from build123d import *
from OCP.BRepFilletAPI import BRepFilletAPI_MakeChamfer

# Parameters (mm, degrees)
SKETCH1_R           = 25
BOSS_EXTRUDE1_DEPTH = 140.711096
SKETCH2_R           = 14.171797432
CUT_EXTRUDE1_DEPTH  = 146.084845995
CHAMFER1_SIZE       = 2.459659
CHAMFER1_SIZE2      = 1.420085


with BuildPart() as part:
    # Sketch1 → Boss-Extrude1 (new body)
    with BuildSketch(Plane(origin=(0, 0, 0), x_dir=(1, 0, 0), z_dir=(0, 1, 0))):
        with Locations(Location((0, 0, 0), (0, 0, 270))):
            Circle(SKETCH1_R)
    extrude(amount=BOSS_EXTRUDE1_DEPTH)

    # Sketch2 → Cut-Extrude1 (cut, through all)
    with BuildSketch(Plane(origin=(0, 0, 0), x_dir=(1, 0, 0), z_dir=(0, 1, 0))):
        with Locations(Location((0, 0, 0), (0, 0, 270))):
            Circle(SKETCH2_R)
    extrude(amount=CUT_EXTRUDE1_DEPTH, mode=Mode.SUBTRACT)

    # Chamfer1: one chamfer whose edges measure the first distance from different faces: ONE call of the kernel's chamfer builder (chamfer() names one face for all edges)
    chamfer1_edges_1 = [part.edges().sort_by_distance(p)[0] for p in [
        (0, 0, -25),
    ]]
    chamfer1_side_1 = [part.faces().sort_by_distance(p)[0] for p in [
        (0, 0, -24.292893219),
    ]]
    chamfer1_edges_2 = [part.edges().sort_by_distance(p)[0] for p in [
        (0, 140.711096, -25),
    ]]
    chamfer1_side_2 = [part.faces().sort_by_distance(p)[0] for p in [
        (0, 70.355548, -25),
    ]]
    chamfer1_edges_3 = [part.edges().sort_by_distance(p)[0] for p in [
        (0, 0, -14.171797432),
    ]]
    chamfer1_side_3 = [part.faces().sort_by_distance(p)[0] for p in [
        (0, 70.355548, -14.171797432),
    ]]
    chamfer1_edges_4 = [part.edges().sort_by_distance(p)[0] for p in [
        (0, 140.711096, -14.171797432),
    ]]
    chamfer1_side_4 = [part.faces().sort_by_distance(p)[0] for p in [
        (0, 140.711096, -24.292893219),
    ]]
    chamfer1 = BRepFilletAPI_MakeChamfer(part.part.solid().wrapped)
    for e in chamfer1_edges_1:
        chamfer1.Add(CHAMFER1_SIZE, CHAMFER1_SIZE2, e.wrapped, chamfer1_side_1[0].wrapped)  # the first distance lies on this face
    for e in chamfer1_edges_2:
        chamfer1.Add(CHAMFER1_SIZE, CHAMFER1_SIZE2, e.wrapped, chamfer1_side_2[0].wrapped)  # the first distance lies on this face
    for e in chamfer1_edges_3:
        chamfer1.Add(CHAMFER1_SIZE, CHAMFER1_SIZE2, e.wrapped, chamfer1_side_3[0].wrapped)  # the first distance lies on this face
    for e in chamfer1_edges_4:
        chamfer1.Add(CHAMFER1_SIZE, CHAMFER1_SIZE2, e.wrapped, chamfer1_side_4[0].wrapped)  # the first distance lies on this face
    add(Compound.cast(chamfer1.Shape()), mode=Mode.REPLACE)


solid = part.part
Here's how the part is built. I have some questions about the finished solid (model axes, mm). Coordinates: 2 decimals unless noted, no trailing zeros. Loops run counter-clockwise (first coordinate to the right, second up) from the corner with the lowest first, then second, coordinate; pieces in that order, holes last.
1. Imagine slicing it at C-C, the plane y = 20.5. Please give me the cut outline in (x, z), and give its area (3 significant figures).
2. Imagine slicing it at A-A, the plane z = 0. Please give me the cut outline in (x, y), and give its area (3 significant figures).
3. I need wall thicknesses on L1, parallel to X at y = 60, z = 0; L2, parallel to X at y = 45, z = 11; L3, parallel to Z at x = 7.5, y = 6. Which ranges of each line are inside material? Lowest first, please.
4. Imagine slicing it at B-B, the plane x = 0. Please give me the cut outline in (y, z).
5. If we mould it in two halves opening along X, with no side actions, what happens to faces 1 (the conical face through (6.82, 0.09, 21.65)), 2 (the conical face through (-13.92, 2.31, -3.09)), 3 (the flat face through (16.1, 140.711, 4.9))? For each: pulls with the +X half, pulls with the -X half, needs draft (parallel to the pull), parting line crosses it, or undercut.
6. For P1, Ø2, axis at x = 15, y = 52, coming from the -Z side; P2, Ø12, axis at x = -15, y = 94.5, coming from the -Z side; P3, Ø4, axis at x = 14, y = 54, coming from the -Z side; P4, Ø4, axis at x = -11, z = -16, coming from the -Y side, each with a flat end and sliding along its axis, tell me the tip position at first contact or that it passes through.
Taken from the geometry:
1. outline: circle Ø50 at (0, 0); hole circle Ø28.34 at (0, 0)
1. area: 1,330 mm2
2. outline: (-25, 1.42) - (-22.54, 0) - (-15.59, 0) - (-14.17, 2.46) - (-14.17, 139.29) - (-16.63, 140.71) - (-23.58, 140.71) - (-25, 138.25) - close; (14.17, 2.46) - (15.59, 0) - (22.54, 0) - (25, 1.42) - (25, 138.25) - (23.58, 140.71) - (16.63, 140.71) - (14.17, 139.29) - close
2. area: 3,030 mm2
3. L1: x = -25 to -14.17, 14.17 to 25
3. L2: x = -22.45 to -8.94, 8.94 to 22.45
3. L3: z = -23.85 to -12.02, 12.02 to 23.85
4. outline: (0, -22.54) - (1.42, -25) - (138.25, -25) - (140.71, -23.58) - (140.71, -16.63) - (139.29, -14.17) - (2.46, -14.17) - (0, -15.59) - close; (0, 15.59) - (2.46, 14.17) - (139.29, 14.17) - (140.71, 16.63) - (140.71, 23.58) - (138.25, 25) - (1.42, 25) - (0, 22.54) - close
5. face 1: parting line crosses it
5. face 2: undercut
5. face 3: needs draft
6. P1: stops at z = -20.71
6. P2: stops at z = -23.32
6. P3: stops at z = -21.93
6. P4: stops at y = 0
